Geometry check sheet. Reference: the model listing, model coordinates, mm. Give positions to 0.01 mm unless a question says otherwise; leave off trailing zeros. Write each loop counter-clockwise with the first axis right and the second up, starting at its lowest first coordinate (ties: lowest second). Pieces come first, ordered by that corner, then holes. Notation, with made-up numbers: (12, 5) -> (70, 5) arc R37 cw to (70, 42) -> close; hole circle Ø3 at (85.5, 18). An arc over 180 degrees is marked (long way). Write item = value, one per line. Start each with the question number.
1. Cross-section at A-A, the plane x = 0. Record the cut outline in (y, z) (3 decimals).
2. Cross-section at C-C, the plane y = 88.5. Record the cut outline in (x, z).
3. Depth check by flat-ended pin: P1, Ø6, axis at x = 7.29, y = -101.35, coming from the -Z side; P2, Ø1, axis at y = -34, z = -2, coming from the -X side; P3, Ø3, axis at y = -60, z = 1, coming from the +X side. Enter the tip coordinate at first touch or a pass-through.
4. Cross-section at B-B, the plane y = -16. Record the cut outline in (x, z).
5. Cross-section at D-D, the plane x = 87. Record the cut outline in (y, z).
6. Thickness scan on line 1 along X through (y, z) = (-1, 0.75); line 2 along Y through (x, z) = (-2, -3.75) (3 decimals); line 3 along X through (y, z) = (14, -1.5). Record the ranges inside material, lowest first.
```python
from build123d import *

# Parameters (mm, degrees)
F0_R      = 106.3498
F1_DEPTH  = 2.116667
F0_R_2    = 107.95
F1_FACE_R = 106.3498
F2_DEPTH  = 2.116667
F3_DEPTH  = 4.233333
F4_R      = 66.675
F5_DEPTH  = 6.351
F6_R      = 3.175
F7_DEPTH  = 25.4
F8_R      = 2.54
F9_DEPTH  = 6.351


with BuildPart() as f1:
    # F0 (on Top) → F1 (new body)
    with BuildSketch(Plane.XY):
        Circle(F0_R)
    extrude(amount=F1_DEPTH)

    # F0 (on Top) + F1_face (on face) → F2 (join)
    with BuildSketch(Plane.XY):
        Circle(F0_R_2)
        Circle(F0_R, mode=Mode.SUBTRACT)
    with BuildSketch(Plane(origin=(0, 0, 0), x_dir=(1, 0, 0), z_dir=(0, 0, -1))):
        Circle(F1_FACE_R)
    extrude(amount=-F2_DEPTH)

    # F0 (on Top) → F3 (join)
    with BuildSketch(Plane.XY):
        Circle(F0_R)
    extrude(amount=-F3_DEPTH)

    # F4 (on face) → F5 (cut, through all)
    with BuildSketch(Plane.XY.offset(2.116667)):
        Circle(F4_R)
    extrude(amount=-F5_DEPTH, mode=Mode.SUBTRACT)

    # F6 (on face) → F7 (cut)
    with BuildSketch(Plane.XY.offset(2.116667)):
        with Locations((-73.088507, -0.004187)):
            Circle(F6_R)
        with Locations((36.448993, 63.237318)):
            Circle(F6_R)
        with Locations((72.961493, -0.004187)):
            Circle(F6_R)
        with Locations((36.448993, -63.245692)):
            Circle(F6_R)
        with Locations((-36.576007, -63.245692)):
            Circle(F6_R)
        with Locations((-36.576007, 63.237318)):
            Circle(F6_R)
    extrude(amount=-F7_DEPTH, mode=Mode.SUBTRACT)

    # F8 (on face) → F9 (cut, through all)
    with BuildSketch(Plane.XY.offset(2.116667)):
        with Locations((-7.293369, -101.353851)):
            Circle(F8_R)
        with Locations((7.293369, -101.353851)):
            Circle(F8_R)
    extrude(amount=-F9_DEPTH, mode=Mode.SUBTRACT)


solid = f1.part
```
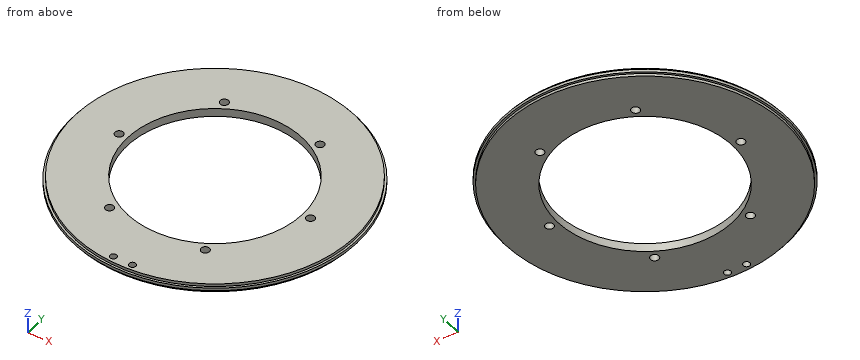
Answers:
q1.outline = (-107.95, -2.117) -> (-106.35, -2.117) -> (-106.35, -4.233) -> (-66.675, -4.233) -> (-66.675, 2.117) -> (-106.35, 2.117) -> (-106.35, 0) -> (-107.95, 0) -> close; (66.675, -4.233) -> (106.35, -4.233) -> (106.35, -2.117) -> (107.95, -2.117) -> (107.95, 0) -> (106.35, 0) -> (106.35, 2.117) -> (66.675, 2.117) -> close
q2.outline = (-61.81, -2.12) -> (-58.97, -2.12) -> (-58.97, -4.23) -> (58.97, -4.23) -> (58.97, -2.12) -> (61.81, -2.12) -> (61.81, 0) -> (58.97, 0) -> (58.97, 2.12) -> (-58.97, 2.12) -> (-58.97, 0) -> (-61.81, 0) -> close
q3.P1 = -4.23
q3.P2 = -102.62
q3.P3 = 90.48
q4.outline = (-106.76, -2.12) -> (-105.14, -2.12) -> (-105.14, -4.23) -> (-64.73, -4.23) -> (-64.73, 2.12) -> (-105.14, 2.12) -> (-105.14, 0) -> (-106.76, 0) -> close; (64.73, -4.23) -> (105.14, -4.23) -> (105.14, -2.12) -> (106.76, -2.12) -> (106.76, 0) -> (105.14, 0) -> (105.14, 2.12) -> (64.73, 2.12) -> close
q5.outline = (-63.91, -2.12) -> (-61.17, -2.12) -> (-61.17, -4.23) -> (61.17, -4.23) -> (61.17, -2.12) -> (63.91, -2.12) -> (63.91, 0) -> (61.17, 0) -> (61.17, 2.12) -> (-61.17, 2.12) -> (-61.17, 0) -> (-63.91, 0) -> close
q6.line_1 = -106.35 to -76.1, -70.07 to -66.67, 66.67 to 69.95, 75.98 to 106.35
q6.line_2 = -106.331 to -66.645, 66.645 to 106.331
q6.line_3 = -107.04 to -65.19, 65.19 to 107.04
